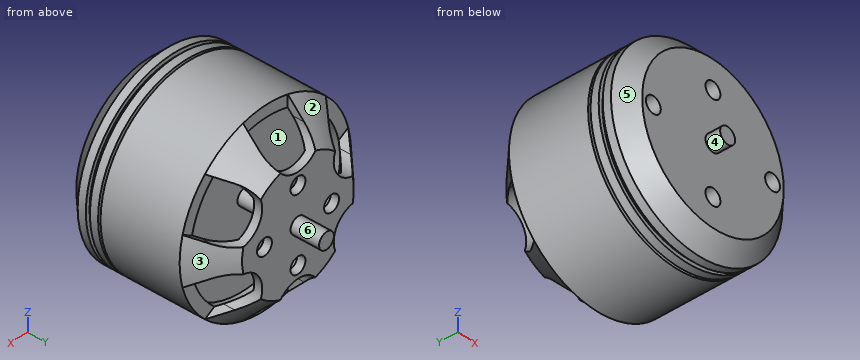
from build123d import *

# Parameters (mm, degrees)
SKETCH2_R          = 1
CUT_EXTRUDE1_DEPTH = 4
SKETCH3_R          = 1
CUT_EXTRUDE2_DEPTH = 3


with BuildPart() as part:
    # Sketch1 → Revolve1 (revolve)
    with BuildSketch(Plane.XY):
        Polygon((0, 0), (0, 21.281896562), (1, 21.281896562), (1, 17.781896562), (7.5, 17.781896562), (11.5, 13.781896562), (11.5, 4.081896562), (9.5, 4.081896562), (9.5, 3.781896562), (11.5, 3.781896562), (11.5, 2.781896562), (11, 2.781896562), (11, 2.281896562), (11.5, 2.281896562), (11.5, 1.281896562), (9.5, -0.718103438), (1, -0.718103438), (1, -2.518103438), (0, -2.518103438), align=None)
        Polygon((2.900417255, 16.781896562), (7.085786438, 16.781896562), (10.5, 13.367683), (10.5, 11.281274074), (1, 11.281274074), (1, 15.781896562), (2.900417255, 15.781896562), align=None, mode=Mode.SUBTRACT)
    revolve(axis=Axis((0, 0, 0), (0, 1, 0)))

    # Sketch2 → Cut-Extrude1 (cut)
    with BuildSketch(Plane(origin=(0, 17.781896562, 0), x_dir=(1, 0, 0), z_dir=(0, 1, 0))):
        with Locations((0, -4.5)):
            Circle(SKETCH2_R)
        with Locations((-4.5, 0)):
            Circle(SKETCH2_R)
        with Locations((0, 4.5)):
            Circle(SKETCH2_R)
        with Locations((4.5, 0)):
            Circle(SKETCH2_R)
        with BuildLine():
            Line((9.294228634, 1.901923789), (15.702595712, 5.601796246))
            Line((15.702595712, 5.601796246), (12.702595712, 10.797948669))
            Line((12.702595712, 10.797948669), (6.294228634, 7.098076211))
            ThreePointArc((6.294228634, 7.098076211), (5.196152423, 3), (9.294228634, 1.901923789))
        make_face()
        with BuildLine():
            Line((-3, 9), (-3, 16.399744914))
            Line((-3, 16.399744914), (3, 16.399744914))
            Line((3, 16.399744914), (3, 9))
            ThreePointArc((3, 9), (0, 6), (-3, 9))
        make_face()
        with BuildLine():
            Line((6.294228634, -7.098076211), (12.702595712, -10.797948669))
            Line((12.702595712, -10.797948669), (15.702595712, -5.601796246))
            Line((15.702595712, -5.601796246), (9.294228634, -1.901923789))
            ThreePointArc((9.294228634, -1.901923789), (5.196152423, -3), (6.294228634, -7.098076211))
        make_face()
        with BuildLine():
            Line((-3, -9), (-3, -16.399744914))
            Line((-3, -16.399744914), (3, -16.399744914))
            Line((3, -16.399744914), (3, -9))
            ThreePointArc((3, -9), (0, -6), (-3, -9))
        make_face()
        with BuildLine():
            Line((-9.294228634, -1.901923789), (-15.702595711, -5.601796246))
            Line((-15.702595711, -5.601796246), (-12.702595711, -10.797948669))
            Line((-12.702595711, -10.797948669), (-6.294228634, -7.098076211))
            ThreePointArc((-6.294228634, -7.098076211), (-5.196152423, -3), (-9.294228634, -1.901923789))
        make_face()
        with BuildLine():
            Line((-6.294228634, 7.098076211), (-12.702595712, 10.797948669))
            Line((-12.702595712, 10.797948669), (-15.702595712, 5.601796246))
            Line((-15.702595712, 5.601796246), (-9.294228634, 1.901923789))
            ThreePointArc((-9.294228634, 1.901923789), (-5.196152423, 3), (-6.294228634, 7.098076211))
        make_face()
    extrude(amount=-CUT_EXTRUDE1_DEPTH, mode=Mode.SUBTRACT)

    # Sketch3 → Cut-Extrude2 (cut)
    with BuildSketch(Plane.XZ.offset(0.718103438)):
        with Locations((8, 0)):
            Circle(SKETCH3_R)
        with Locations((-8, 0)):
            Circle(SKETCH3_R)
        with Locations((0, 6)):
            Circle(SKETCH3_R)
        with Locations((0, -6)):
            Circle(SKETCH3_R)
    extrude(amount=-CUT_EXTRUDE2_DEPTH, mode=Mode.SUBTRACT)


solid = part.part
CAD build for the part. Positions are in the model's coordinates, mm. Face numbers are marked on the shaded views. A direction names the side the tool comes from. Coordinates: 2 decimals unless noted, no trailing zeros. Answer as a JSON object with one key per item and string values. Group by question number.
1) Mould opens along X. For the marked faces 1, 2, 3 and 4 say: +X half, -X half, draft (parallel to the pull), parting line (faces both ways), or undercut.
2) Pin check, flat tips, straight feed: pin 1 Ø1.6 at (x, z) = (0, 4.5) entering from -Y; pin 2 Ø12 at (x, y) = (-6.5, 18) entering from +Z; pin 3 Ø3 at (x, y) = (-4.5, 0.5) entering from +Z. Stop position of each tip, or through.
3) Saw through at A-A (z = 4.5). Give the number of separate pieces and of enclosed holes in the cut face, plus the area to 3 significant figures.
4) Tool access for the marked faces 5 and 6: list every direction of +Z, -Z, +X, -X, +Y, -Y with a clear straight run to the whole face (end or side of a thin tool).
5) Wall check: line 1 (Z direction, x = 0, y = 12.35); line 2 (Y direction, x = 3.75, z = -2.5); line 3 (X direction, y = 17.45, z = 4.5). Give the ranges that are in metal, low to high. Write a range as from..to.
Values follow:
{
 "1": {"face 1": "undercut", "face 2": "-X half", "face 3": "+X half", "face 4": "parting line"},
 "2": {"pin 1": "stops at y = -0.72", "pin 2": "stops at z = 11.28", "pin 3": "stops at z = 11.04"},
 "3": {"separate pieces": "3", "enclosed holes": "0", "area": "261 mm2"},
 "4": {"face 5": "-Y", "face 6": "+Y"},
 "5": {"line 1": "z = -11.5..-10.5, -1..1, 10.5..11.5", "line 2": "y = -0.72..11.28, 16.78..17.78", "line 3": "x = -4.79..-1, 1..4.79"}
}
